The model under review builds one solid part; all positions refer to its coordinate system, in mm. A direction names the side the tool comes from. Round coordinates to 2 decimals unless told otherwise and drop trailing zeros. Write each loop counter-clockwise with the first axis right and the second up, starting at its lowest first coordinate (ties: lowest second). Pieces come first, ordered by that corner, then holes. Notation, with made-up numbers: M 85.5,-25 L 102.5,-25 A28 cw 102.5,1 Z; hole C -11.5,52 d10. An arc over 180 degrees is marked long. Write item = value, one per line. Start each with the question number.
Item 1: Take a section at D-D, the plane y = 1. Give the boundary of the cut face in (x, z).
Item 2: To check wall thickness, follow line 1 along Y through (x, z) = (6, 6.5); line 2 along X through (y, z) = (-2.25, 3); line 3 along Z through (x, y) = (-2, -3.5). State the ranges of each line that lie inside material, in increasing order.
Item 3: Take a section at A-A, the plane z = 6. Give the boundary of the cut face in (x, y).
Item 4: Take a section at C-C, the plane x = 3.81. Give the boundary of the cut face in (y, z).
Item 5: Tool access review of faces 1 (the flat face through (-14.554, 0, 4)), 2 (the cylindrical face through (-2.67, -1.743, 10.49)), 3 (the flat face through (12, 4, 11.455)): name each direction out of +Z, -Z, +X, -X, +Y, -Y from which nothing blocks a thin tool from reaching the whole face with its end or side.
Item 6: The part is to be moulded in two halves that separate along X. For faces 4 (the flat face through (-1, -7, 0)), 5 (the flat face through (-15.888, 0, 5)), 6 (the flat face through (14.554, 0, 4)), 7 (the flat face through (0, 0, 7.62)), say which applies: +X half, -X half, draft (parallel to the pull), parting line (faces both ways), or undercut.
Item 7: Take a section at B-B, the plane y = 3.81. Give the boundary of the cut face in (x, z), plus the area to 3 significant figures.
Item 8: For pin 1 Ø2 at (x, y) = (-4.5, 2) entering from -Z, flat-tipped, find the tip position at first contact; note if it passes through.
from build123d import *

# Parameters (mm, degrees)
F0_W      = 31.7754
F0_H      = 15.8242
F1_DEPTH  = 9.5504
F2_R      = 2.4511
F4_DEPTH  = 1.905
F3_R      = 2.4511
F5_DEPTH  = 1.905
F6_R      = 2.4511
F8_DEPTH  = 1.905
F7_R      = 2.4511
F9_DEPTH  = 1.905
F10_R     = 2.4511
F11_DEPTH = 1.905
F12_R     = 2.4511
F13_DEPTH = 1.905
F14_W     = 29.1084
F14_H     = 13.3858
F15_DEPTH = 7.62


with BuildPart() as f1:
    # F0 (on Top) → F1 (new body)
    with BuildSketch(Plane.XY):
        Rectangle(F0_W, F0_H)
    extrude(amount=F1_DEPTH)

    # F2 (on face) → F4 (join)
    with BuildSketch(Plane.XY.offset(9.5504)):
        with Locations((-11.7856, 3.81)):
            Circle(F2_R)
    extrude(amount=F4_DEPTH)

    # F3 (on face) → F5 (join)
    with BuildSketch(Plane.XY.offset(9.5504)):
        with Locations((-11.7856, -3.81)):
            Circle(F3_R)
    extrude(amount=F5_DEPTH)

    # F6 (on face) → F8 (join)
    with BuildSketch(Plane.XY.offset(9.5504)):
        with Locations((-3.9878, 3.81)):
            Circle(F6_R)
    extrude(amount=F8_DEPTH)

    # F7 (on face) → F9 (join)
    with BuildSketch(Plane.XY.offset(9.5504)):
        with Locations((-3.9878, -3.81)):
            Circle(F7_R)
    extrude(amount=F9_DEPTH)

    # F10 (on face) → F11 (join)
    with BuildSketch(Plane.XY.offset(9.5504)):
        with Locations((3.81, 3.81)):
            Circle(F10_R)
        with Locations((3.81, -3.81)):
            Circle(F10_R)
    extrude(amount=F11_DEPTH)

    # F12 (on face) → F13 (join)
    with BuildSketch(Plane.XY.offset(9.5504)):
        with Locations((11.6078, 3.81)):
            Circle(F12_R)
        with Locations((11.6078, -3.81)):
            Circle(F12_R)
    extrude(amount=F13_DEPTH)

    # F14 (on face) → F15 (cut)
    with BuildSketch(Plane(origin=(0, 0, 0), x_dir=(1, 0, 0), z_dir=(0, 0, -1))):
        Rectangle(F14_W, F14_H)
    extrude(amount=-F15_DEPTH, mode=Mode.SUBTRACT)


solid = f1.part
Response values:
q1.outline = M -15.89,0 L -14.55,0 L -14.55,7.62 L 14.55,7.62 L 14.55,0 L 15.89,0 L 15.89,9.55 L -15.89,9.55 Z
q2.line_1 = -7.91 to -6.69, 6.69 to 7.91
q2.line_2 = -15.89 to -14.55, 14.55 to 15.89
q2.line_3 = 7.62 to 11.46
q3.outline = M -15.89,-7.91 L 15.89,-7.91 L 15.89,7.91 L -15.89,7.91 Z; hole M -14.55,-6.69 L 14.55,-6.69 L 14.55,6.69 L -14.55,6.69 Z
q4.outline = M -7.91,0 L -6.69,0 L -6.69,7.62 L 6.69,7.62 L 6.69,0 L 7.91,0 L 7.91,9.55 L 6.26,9.55 L 6.26,11.46 L 1.36,11.46 L 1.36,9.55 L -1.36,9.55 L -1.36,11.46 L -6.26,11.46 L -6.26,9.55 L -7.91,9.55 Z
q5.face_1 = -Z
q5.face_2 = +Z
q5.face_3 = +Z, +X, -X, +Y, -Y
q6.face_4 = draft
q6.face_5 = -X half
q6.face_6 = undercut
q6.face_7 = undercut
q7.outline = M -15.89,0 L -14.55,0 L -14.55,7.62 L 14.55,7.62 L 14.55,0 L 15.89,0 L 15.89,9.55 L 14.06,9.55 L 14.06,11.46 L 9.16,11.46 L 9.16,9.55 L 6.26,9.55 L 6.26,11.46 L 1.36,11.46 L 1.36,9.55 L -1.54,9.55 L -1.54,11.46 L -6.44,11.46 L -6.44,9.55 L -9.33,9.55 L -9.33,11.46 L -14.24,11.46 L -14.24,9.55 L -15.89,9.55 Z
q7.area = 119 mm2
q8.pin_1 = 7.62
